```python
from build123d import *
from OCP.BRepFilletAPI import BRepFilletAPI_MakeChamfer

# Parameters (mm, degrees)
RESSALTO_EXTRUS_O1_DEPTH    = 8
CORTE_EXTRUS_O1_START       = -8
CORTE_EXTRUS_O1_OUTLINE_W   = 7
CORTE_EXTRUS_O1_OUTLINE_H   = 12
CORTE_EXTRUS_O1_OUTLINE_W_2 = 6
CORTE_EXTRUS_O1_OUTLINE_H_2 = 8.6
CORTE_EXTRUS_O1_DEPTH       = 8
CORTE_EXTRUS_O2_DEPTH       = 16.099668871
CORTE_EXTRUS_O2_DEPTH_BACK  = 16.099668871
ESBO_O3_W                   = 8.6
ESBO_O3_H                   = 5
CORTE_EXTRUS_O3_DEPTH       = 18.756407294
CORTE_EXTRUS_O3_DEPTH_BACK  = 18.756407294
ESBO_O4_R                   = 1.65
ESBO_O5_R                   = 1.5
RESSALTO_EXTRUS_O2_DEPTH    = 1.5
FILETE1_R                   = 2
CHANFRO1_SIZE               = 0.8
CHANFRO1_SIZE2              = 0.461880215
ESBO_O7_W                   = 9.300626083
ESBO_O7_H                   = 16
CORTE_EXTRUS_O5_DEPTH       = 10
RESSALTO_EXTRUS_O4_DEPTH    = 7
ESBO_O10_R                  = 1.65
CORTE_EXTRUS_O6_DEPTH       = 18.895530168
CHANFRO2_SIZE               = 3


# Read off the part's stored shape, not the designer's step: Corte-extrusão1
with BuildPart() as part:
    # Esboço1 → Ressalto-extrusão1 (new, symmetric)
    with BuildSketch(Plane.XY):
        with BuildLine():
            Line((-6, 0), (6, 0))
            Line((6, 0), (6, -5.690598923))
            Line((6, -5.690598923), (2, -8))
            Line((2, -8), (-6, -8))
            ThreePointArc((-6, -8), (-10, -4), (-6, 0))
        make_face()
    extrude(amount=RESSALTO_EXTRUS_O1_DEPTH, both=True)

    # Corte-extrusão1 outline → Corte-extrusão1 (cut)
    with BuildSketch(Plane(origin=(0, 0, 0), x_dir=(1, 0, 0), z_dir=(0, 1, 0)).offset(CORTE_EXTRUS_O1_START)):
        with Locations((-6.5, 0)):
            Rectangle(CORTE_EXTRUS_O1_OUTLINE_W, CORTE_EXTRUS_O1_OUTLINE_H)
        with Locations((3, 0)):
            Rectangle(CORTE_EXTRUS_O1_OUTLINE_W_2, CORTE_EXTRUS_O1_OUTLINE_H_2)
    extrude(amount=CORTE_EXTRUS_O1_DEPTH, mode=Mode.SUBTRACT)

    # Esboço3 → Corte-extrusão2 (cut, two sides: drawn at the far end of the back side and taken through both)
    with BuildSketch(Plane(origin=(0, 0, 0), x_dir=(0, 0, -1), z_dir=(1, 0, 0)).offset(-CORTE_EXTRUS_O2_DEPTH_BACK)):
        with Locations((0, -4)):
            Rectangle(ESBO_O3_W, ESBO_O3_H)
    extrude(amount=CORTE_EXTRUS_O2_DEPTH + CORTE_EXTRUS_O2_DEPTH_BACK, mode=Mode.SUBTRACT)

    # Esboço4 → Corte-extrusão3 (cut, two sides: drawn at the far end of the back side and taken through both)
    with BuildSketch(Plane(origin=(0, 0, 4.3), x_dir=(-1, 0, 0), z_dir=(0, 0, -1)).offset(-CORTE_EXTRUS_O3_DEPTH_BACK)):
        with Locations((-3.2, -4)):
            Circle(ESBO_O4_R)
    extrude(amount=CORTE_EXTRUS_O3_DEPTH + CORTE_EXTRUS_O3_DEPTH_BACK, mode=Mode.SUBTRACT)

    # Esboço5 → Ressalto-extrusão2 (add)
    with BuildSketch(Plane(origin=(0, 0, 6), x_dir=(-1, 0, 0), z_dir=(0, 0, -1))):
        with Locations((6, -4)):
            Circle(ESBO_O5_R)
    ressalto_extrus_o2 = extrude(amount=RESSALTO_EXTRUS_O2_DEPTH)

    # Espelhar1: Ressalto-extrusão2 across plane
    add(ressalto_extrus_o2.mirror(Plane.XY))

    # Filete1
    filete1_edges = [part.edges().sort_by_distance(p)[0] for p in [
        (6, -5.690598923, -6.15),
        (6, -5.690598923, 6.15),
    ]]
    fillet(filete1_edges, radius=FILETE1_R)

    # Chanfro1: one chamfer whose edges measure the first distance from different faces: ONE call of the kernel's chamfer builder (chamfer() names one face for all edges)
    chanfro1_edges_1 = [part.edges().sort_by_distance(p)[0] for p in [
        (-4.5, -4, 4.5),
    ]]
    chanfro1_side_1 = [part.faces().sort_by_distance(p)[0] for p in [
        (-4.5, -4, 5.25),
    ]]
    chanfro1_edges_2 = [part.edges().sort_by_distance(p)[0] for p in [
        (-4.5, -4, -4.5),
    ]]
    chanfro1_side_2 = [part.faces().sort_by_distance(p)[0] for p in [
        (-4.5, -4, -5.25),
    ]]
    chanfro1_edges_3 = [part.edges().sort_by_distance(p)[0] for p in [
        (4.85, -4, -4.3),
    ]]
    chanfro1_side_3 = [part.faces().sort_by_distance(p)[0] for p in [
        (4.85, -4, -6.15),
    ]]
    chanfro1_edges_4 = [part.edges().sort_by_distance(p)[0] for p in [
        (4.85, -4, 4.3),
    ]]
    chanfro1_side_4 = [part.faces().sort_by_distance(p)[0] for p in [
        (4.85, -4, 6.15),
    ]]
    chanfro1 = BRepFilletAPI_MakeChamfer(part.part.solid().wrapped)
    for e in chanfro1_edges_1:
        chanfro1.Add(CHANFRO1_SIZE, CHANFRO1_SIZE2, e.wrapped, chanfro1_side_1[0].wrapped)  # the first distance lies on this face
    for e in chanfro1_edges_2:
        chanfro1.Add(CHANFRO1_SIZE, CHANFRO1_SIZE2, e.wrapped, chanfro1_side_2[0].wrapped)  # the first distance lies on this face
    for e in chanfro1_edges_3:
        chanfro1.Add(CHANFRO1_SIZE, CHANFRO1_SIZE2, e.wrapped, chanfro1_side_3[0].wrapped)  # the first distance lies on this face
    for e in chanfro1_edges_4:
        chanfro1.Add(CHANFRO1_SIZE, CHANFRO1_SIZE2, e.wrapped, chanfro1_side_4[0].wrapped)  # the first distance lies on this face
    add(Compound.cast(chanfro1.Shape()), mode=Mode.REPLACE)

    # Esboço7 → Corte-extrusão5 (cut)
    with BuildSketch(Plane(origin=(0, 0, 0), x_dir=(1, 0, 0), z_dir=(0, 1, 0))):
        with Locations((4.650313042, 0)):
            Rectangle(ESBO_O7_W, ESBO_O7_H)
    extrude(amount=-CORTE_EXTRUS_O5_DEPTH, mode=Mode.SUBTRACT)

    # Esboço9 → Ressalto-extrusão4 (add, symmetric)
    with BuildSketch(Plane.XY):
        Polygon((0, -8), (0, -10.5), (10, -10.5), (10, -12.5), (-3, -12.5), (-3, -8), align=None)
    extrude(amount=RESSALTO_EXTRUS_O4_DEPTH, both=True)

    # Esboço10 → Corte-extrusão6 (cut, through all)
    with BuildSketch(Plane(origin=(0, 0, 0), x_dir=(1, 0, 0), z_dir=(0, 1, 0))):
        with Locations(Location((6, 0.5, 0), (0, 0, 180))):
            Circle(ESBO_O10_R)
        Polygon((6, 6.5), (10, 2.5), (10, 8), (5.06809326, 8), (0, 8), (0, 6.5), align=None)
        Polygon((10, -1.5), (6, -5.5), (0, -5.5), (0, -8), (10, -8), align=None)
    extrude(amount=-CORTE_EXTRUS_O6_DEPTH, mode=Mode.SUBTRACT)

    # Chanfro2
    chanfro2_edges = [part.edges().sort_by_distance(p)[0] for p in [
        (0, -10.5, -0.5),
    ]]
    chamfer(chanfro2_edges, length=CHANFRO2_SIZE)


solid = part.part
```
Read the model definition and answer for the solid it produces. Units are mm, in the model's axes. A direction names the side the tool comes from. Round coordinates to 2 decimals unless told otherwise and drop trailing zeros. Write each loop counter-clockwise with the first axis right and the second up, starting at its lowest first coordinate (ties: lowest second). Pieces come first, ordered by that corner, then holes. Notation, with made-up numbers: (84, 5.25) - (116, 5.25) arc R20 ccw to (116, 37.25) - close; hole circle Ø6 at (40, -10.75). An arc over 180 degrees is marked (long way). Use CSV: the item, a comma, the result in double quotes.
Q1. A tool of negligible diameter and unlimited length cuts with its end or side. For faces 4 (the flat face through (-1, -10, 7)), 5 (the flat face through (5, -10.5, -2)), 6 (the flat face through (-6, -4, -4.5)), from which of +Z, -Z, +X, -X, +Y, -Y can it reach the whole face along a straight path? Write none if from no direction.
Values:
face 4,"+Z, +X, -X, -Y"
face 5,"+Z, -Z, +X, +Y"
face 6,"-X, +Y, -Y"
Q2. Each of these flat-tipped pins is pushed along its axis until it touches: pin 1 Ø1.6 at (x, z) = (-3.5, 7) entering from -Y; pin 2 Ø2 at (x, z) = (8, -3) entering from +Y; pin 3 Ø0.9 at (x, y) = (-2, -9) entering from -Z; pin 4 Ø2 at (y, z) = (-7, -4) entering from +X. Where does it stop, or does it pass through?
Values:
pin 1,"stops at y = -12.5"
pin 2,"stops at y = -10.5"
pin 3,"stops at z = -7"
pin 4,"stops at x = 0.5"
Q3. Find section B-B, the plane z = 2.75. Write down the section's boundary in (x, y).
Values:
outline,"(-3, -12.5) - (8.75, -12.5) - (8.75, -10.5) - (3, -10.5) - (0, -7.5) - (0, -6.5) - (-3, -6.5) - close; (-3, -1.5) - (0, -1.5) - (0, 0) - (-3, 0) - close"
Q4. Find section D-D, the plane z = -0.5. Write down the section's boundary in (x, y).
Values:
outline,"(-3, -12.5) - (4.35, -12.5) - (4.35, -10.5) - (3, -10.5) - (0, -7.5) - (0, -6.5) - (-3, -6.5) - close; (-3, -1.5) - (0, -1.5) - (0, 0) - (-3, 0) - close; (7.65, -12.5) - (10, -12.5) - (10, -10.5) - (7.65, -10.5) - close"
Q5. Find section A-A, the plane y = -4. Write down the section's boundary in (x, z).
Values:
outline,"(-10, -8) - (0, -8) - (0, -4.3) - (-3, -4.3) - (-3, -6) - (-4.5, -6) - (-4.5, -5.3) - (-4.96, -4.5) - (-7.04, -4.5) - (-7.5, -5.3) - (-7.5, -6) - (-10, -6) - close; (-10, 6) - (-7.5, 6) - (-7.5, 5.3) - (-7.04, 4.5) - (-4.96, 4.5) - (-4.5, 5.3) - (-4.5, 6) - (-3, 6) - (-3, 4.3) - (0, 4.3) - (0, 8) - (-10, 8) - close"
Q6. Straight lines are drawn through the part: line 1 along Z through (x, y) = (-0.5, -3.75); line 2 along Z through (x, y) = (-4.25, -7.75); line 3 along Y through (x, z) = (-2.75, 0.75). For each, find the intervals that lie inside material, in ascending order.
Values:
line 1,"z = -8 to -4.3, 4.3 to 8"
line 2,"z = -8 to -6, 6 to 8"
line 3,"y = -12.5 to -6.5, -1.5 to 0"
Q7. Determine the mould class of faces 1 (the flat face through (-1, -10, -7)), 2 (the flat face through (-3, -8, 0)), 3 (the flat face through (10, -11, 0)) for opening direction Z: +Z half, -Z half, draft (parallel to the pull), parting line (faces both ways), or undercut.
Values:
face 1,"-Z half"
face 2,"undercut"
face 3,"draft"
Q8. Find section C-C, the plane x = -1.75. Write down the section's boundary in (y, z).
Values:
outline,"(-12.5, -7) - (-8, -7) - (-8, -8) - (0, -8) - (0, 8) - (-8, 8) - (-8, 7) - (-12.5, 7) - close; hole (-6.5, -4.3) - (-1.5, -4.3) - (-1.5, 4.3) - (-6.5, 4.3) - close"
